```python
from build123d import *

# Parameters (mm, degrees)
SKETCH6_W           = 127
SKETCH6_H           = 50.8
SKETCH6_R           = 2.5527
BOSS_EXTRUDE1_DEPTH = 6.35
FILLET1_R           = 6.35


with BuildPart() as part:
    # Sketch6 → Boss-Extrude1 (new body)
    with BuildSketch(Plane.XY):
        Rectangle(SKETCH6_W, SKETCH6_H)
        with Locations((-50.8, 0)):
            Circle(SKETCH6_R, mode=Mode.SUBTRACT)
        with Locations((-50.8, 12.7)):
            Circle(SKETCH6_R, mode=Mode.SUBTRACT)
        with Locations((-50.8, -12.7)):
            Circle(SKETCH6_R, mode=Mode.SUBTRACT)
        with Locations((-38.1, -12.7)):
            Circle(SKETCH6_R, mode=Mode.SUBTRACT)
        with Locations((-38.1, 0)):
            Circle(SKETCH6_R, mode=Mode.SUBTRACT)
        with Locations((-38.1, 12.7)):
            Circle(SKETCH6_R, mode=Mode.SUBTRACT)
        with Locations((-25.4, -12.7)):
            Circle(SKETCH6_R, mode=Mode.SUBTRACT)
        with Locations((-25.4, 0)):
            Circle(SKETCH6_R, mode=Mode.SUBTRACT)
        with Locations((-25.4, 12.7)):
            Circle(SKETCH6_R, mode=Mode.SUBTRACT)
        with Locations((-12.7, -12.7)):
            Circle(SKETCH6_R, mode=Mode.SUBTRACT)
        with Locations((-12.7, 0)):
            Circle(SKETCH6_R, mode=Mode.SUBTRACT)
        with Locations((-12.7, 12.7)):
            Circle(SKETCH6_R, mode=Mode.SUBTRACT)
        with Locations((0, -12.7)):
            Circle(SKETCH6_R, mode=Mode.SUBTRACT)
        Circle(SKETCH6_R, mode=Mode.SUBTRACT)
        with Locations((0, 12.7)):
            Circle(SKETCH6_R, mode=Mode.SUBTRACT)
        with Locations((12.7, -12.7)):
            Circle(SKETCH6_R, mode=Mode.SUBTRACT)
        with Locations((12.7, 0)):
            Circle(SKETCH6_R, mode=Mode.SUBTRACT)
        with Locations((12.7, 12.7)):
            Circle(SKETCH6_R, mode=Mode.SUBTRACT)
        with Locations((25.4, -12.7)):
            Circle(SKETCH6_R, mode=Mode.SUBTRACT)
        with Locations((25.4, 0)):
            Circle(SKETCH6_R, mode=Mode.SUBTRACT)
        with Locations((25.4, 12.7)):
            Circle(SKETCH6_R, mode=Mode.SUBTRACT)
        with Locations((38.1, -12.7)):
            Circle(SKETCH6_R, mode=Mode.SUBTRACT)
        with Locations((38.1, 0)):
            Circle(SKETCH6_R, mode=Mode.SUBTRACT)
        with Locations((38.1, 12.7)):
            Circle(SKETCH6_R, mode=Mode.SUBTRACT)
        with Locations((50.8, -12.7)):
            Circle(SKETCH6_R, mode=Mode.SUBTRACT)
        with Locations((50.8, 0)):
            Circle(SKETCH6_R, mode=Mode.SUBTRACT)
        with Locations((50.8, 12.7)):
            Circle(SKETCH6_R, mode=Mode.SUBTRACT)
    extrude(amount=BOSS_EXTRUDE1_DEPTH)

    # Fillet1
    fillet1_edges = [part.edges().sort_by_distance(p)[0] for p in [
        (63.5, -25.4, 3.175),
        (-63.5, -25.4, 3.175),
        (-63.5, 25.4, 3.175),
        (63.5, 25.4, 3.175),
    ]]
    fillet(fillet1_edges, radius=FILLET1_R)


solid = part.part
```
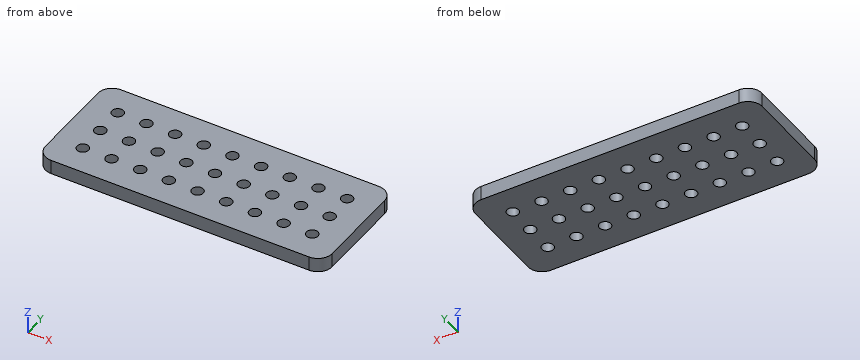
Read the model definition and answer for the solid it produces. Units are mm, in the model's axes. Round coordinates to 2 decimals unless told otherwise and drop trailing zeros. Write each loop counter-clockwise with the first axis right and the second up, starting at its lowest first coordinate (ties: lowest second). Pieces come first, ordered by that corner, then holes. Notation, with made-up numbers: M 35,21.25 L 75,21.25 A29 ccw 75,44.25 Z; hole C 55,86.25 d3. An arc over 180 degrees is marked long. One line per item, written item: value.
Q1. Find section A-A on x = 12.7. Write down the section's boundary in (y, z), plus the area to 3 significant figures.
Data:
outline: M -25.4,0 L -15.25,0 L -15.25,6.35 L -25.4,6.35 Z; M -10.15,0 L -2.55,0 L -2.55,6.35 L -10.15,6.35 Z; M 2.55,0 L 10.15,0 L 10.15,6.35 L 2.55,6.35 Z; M 15.25,0 L 25.4,0 L 25.4,6.35 L 15.25,6.35 Z
area: 225 mm2
Q2. Straight lines are drawn through the part: line 1 (Y direction, x = 25.4, z = 3.25); line 2 (Y direction, x = -39.5, z = 1.5); line 3 (X direction, y = -19.5, z = 5.5). For each, find the intervals that lie inside material, in ascending order. Write a range as [from, to].
Data:
line 1: [-25.4, -15.25], [-10.15, -2.55], [2.55, 10.15], [15.25, 25.4]
line 2: [-25.4, -14.83], [-10.57, -2.13], [2.13, 10.57], [14.83, 25.4]
line 3: [-63.48, 63.48]
Q3. Find section B-B on z = 4.25. Count the separate pieces of the cut face and the enclosed holes in it, plus the area to 3 significant figures.
Data:
separate pieces: 1
enclosed holes: 27
area: 5,860 mm2
Q4. Find section D-D on x = -1. Write down the section's boundary in (y, z).
Data:
outline: M -25.4,0 L -15.05,0 L -15.05,6.35 L -25.4,6.35 Z; M -10.35,0 L -2.35,0 L -2.35,6.35 L -10.35,6.35 Z; M 2.35,0 L 10.35,0 L 10.35,6.35 L 2.35,6.35 Z; M 15.05,0 L 25.4,0 L 25.4,6.35 L 15.05,6.35 Z
